from build123d import *

# Parameters (mm, degrees)
SKETCH1_W                        = 76.2
SKETCH1_H                        = 925.5125
BASE_FLANGE1_DEPTH               = 3.175
EDGE_FLANGE1_STRIP_W             = 20.32
EDGE_FLANGE1_STRIP_H             = 3.175
EDGE_FLANGE1_STRIP_CUT_DEPTH     = 925.5125
EDGE_FLANGE1_DEPTH               = 925.5125
EDGE_FLANGE2_STRIP_W             = 20.32
EDGE_FLANGE2_STRIP_H             = 3.175
EDGE_FLANGE2_STRIP_CUT_DEPTH     = 925.5125
EDGE_FLANGE2_DEPTH               = 925.5125
F_10_0_1935_DIAMETER_HOLE2_D     = 4.9149
F_10_0_1935_DIAMETER_HOLE1_D     = 4.9149
FILLET1_R                        = 3.175
O_0_316_DIAMETER_HOLE1_D         = 8.0264
F_27_64_0_42188_DIAMETER_HOLE1_D = 10.715752


# Sheet-metal steps are written as plain solids
with BuildPart() as part:
    # Sketch1 → Base-Flange1 (new body)
    with BuildSketch(Plane(origin=(0, 0, 0), x_dir=(0, 0, -1), z_dir=(1, 0, 0))):
        with Locations((38.1, 462.75625)):
            Rectangle(SKETCH1_W, SKETCH1_H)
    extrude(amount=-BASE_FLANGE1_DEPTH)

    # Edge-Flange1 strip (across the edge) → Edge-Flange1 strip cut (cut)
    with BuildSketch(Plane(origin=(-3.175, 0, 0), x_dir=(0, 0, -1), z_dir=(0, 1, 0))):
        with Locations((-6.35, -1.5875)):
            Rectangle(EDGE_FLANGE1_STRIP_W, EDGE_FLANGE1_STRIP_H)
    extrude(amount=EDGE_FLANGE1_STRIP_CUT_DEPTH, mode=Mode.SUBTRACT)

    # Edge-Flange1 section (across the edge) → Edge-Flange1 (add)
    with BuildSketch(Plane(origin=(-3.175, 0, 0), x_dir=(0, 0, -1), z_dir=(0, 1, 0))):
        with BuildLine():
            Line((-3.175, 3.81), (-3.175, 53.975))
            Line((-3.175, 53.975), (0, 53.975))
            Line((0, 53.975), (0, 3.81))
            ThreePointArc((0, 3.81), (1.115923164, 1.115923164), (3.81, 0))
            Line((3.81, 0), (3.81, -3.175))
            ThreePointArc((3.81, -3.175), (-1.129140867, -1.129140867), (-3.175, 3.81))
        make_face()
    extrude(amount=EDGE_FLANGE1_DEPTH)

    # Edge-Flange2 strip (across the edge) → Edge-Flange2 strip cut (cut)
    with BuildSketch(Plane(origin=(-3.175, 925.5125, -76.2), x_dir=(0, 0, 1), z_dir=(0, -1, 0))):
        with Locations((-6.35, -1.5875)):
            Rectangle(EDGE_FLANGE2_STRIP_W, EDGE_FLANGE2_STRIP_H)
    extrude(amount=EDGE_FLANGE2_STRIP_CUT_DEPTH, mode=Mode.SUBTRACT)

    # Edge-Flange2 section (across the edge) → Edge-Flange2 (add)
    with BuildSketch(Plane(origin=(-3.175, 925.5125, -76.2), x_dir=(0, 0, 1), z_dir=(0, -1, 0))):
        with BuildLine():
            Line((-3.175, 3.81), (-3.175, 53.975))
            Line((-3.175, 53.975), (0, 53.975))
            Line((0, 53.975), (0, 3.81))
            ThreePointArc((0, 3.81), (1.115923164, 1.115923164), (3.81, 0))
            Line((3.81, 0), (3.81, -3.175))
            ThreePointArc((3.81, -3.175), (-1.129140867, -1.129140867), (-3.175, 3.81))
        make_face()
    extrude(amount=EDGE_FLANGE2_DEPTH)

    # #10 (0.1935) Diameter Hole2 (through all)
    with Locations(Plane(origin=(0, 0, -79.375), x_dir=(-1, 0, 0), z_dir=(0, 0, -1))):
        with Locations((20.6375, 19.05), (46.0375, 19.05)):
            Hole(F_10_0_1935_DIAMETER_HOLE2_D / 2)

    # #10 (0.1935) Diameter Hole1 (through all)
    with Locations(Plane(origin=(0, 0, -79.375), x_dir=(-1, 0, 0), z_dir=(0, 0, -1))):
        with Locations((46.0375, 912.8125), (20.6375, 912.8125), (20.6375, 887.4125), (46.0375, 887.4125)):
            Hole(F_10_0_1935_DIAMETER_HOLE1_D / 2)

    # Fillet1
    fillet1_edges = [part.edges().sort_by_distance(p)[0] for p in [
        (-57.15, 0, 1.5875),
        (-57.15, 925.5125, 1.5875),
        (-57.15, 925.5125, -77.7875),
        (-57.15, 0, -77.7875),
    ]]
    fillet(fillet1_edges, radius=FILLET1_R)

    # O (0.316) Diameter Hole1 (through all)
    with Locations(Plane(origin=(0, 0, -79.375), x_dir=(-1, 0, 0), z_dir=(0, 0, -1))):
        with Locations((14.2875, 520.7), (14.2875, 444.5), (46.0375, 520.7), (46.0375, 444.5)):
            Hole(O_0_316_DIAMETER_HOLE1_D / 2)

    # 27/64 (0.42188) Diameter Hole1 (through all)
    with Locations(Plane.XY.offset(3.175)):
        with Locations((-41.275, 825.5), (-41.275, 781.05), (-41.275, 628.65), (-41.275, 584.2)):
            Hole(F_27_64_0_42188_DIAMETER_HOLE1_D / 2)


solid = part.part
Can you work these out from the model? Positions are in its coordinate system, mm. A direction names the side the tool comes from. Give positions to 0.01 mm unless a question says otherwise; leave off trailing zeros. Write each loop counter-clockwise with the first axis right and the second up, starting at its lowest first coordinate (ties: lowest second). Pieces come first, ordered by that corner, then holes. Notation, with made-up numbers: (31, -20.5) -> (46, -20.5) arc R24 ccw to (46, 14.5) -> close; hole circle Ø11 at (-3.5, -37). An arc over 180 degrees is marked (long way). Answer as a JSON object with one key per item and string values. Group by question number.
Item 1: Suppose I cut it at A-A (y = 290.5). Please give me the cut outline in (x, z) (3 decimals), plus the area to 3 significant figures.
Item 2: Suppose I cut it at B-B (z = -37). Please give me the cut outline in (x, y) (1 decimal), plus the area to 3 significant figures.
Item 3: I'm going to push flat-ended pins straight in: P1, Ø12, axis at y = 102.5, z = -41.5, coming from the -X side (3 decimals); P2, Ø9.5, axis at x = -41.275, y = 628.65, coming from the -Z side. Where does each tip first touch, or does it pass through?
Item 4: We'd pull the mould along Z, two halves only. Please class faces 3 (the face through (-3, 0, -38)), 4 (the face through (-32, 456, 3.175)), 5 (the face through (-3.175, 469, -38)), 6 (the face through (-32, 469, -79.375)): +Z half, -Z half, draft (parallel to the pull), parting line (faces both ways), or undercut.
Item 5: For faces 1 (the face through (-3, 925.512, -38)), 2 (the face through (-32, 456, 0)), which set-ups out of +Z, -Z, +X, -X, +Y, -Y let a thin tool reach every point of the face, with its end or its side?
Item 6: Please list where these lines run through material, in increasing order: line 1 (X direction, y = 444.5, z = 2.1); line 2 (Z direction, x = -20, y = 554.5) (3 decimals); line 3 (X direction, y = 324.5, z = -34) (3 decimals). Write a range as [from, to].
Findings:
{
 "1": {"outline": "(-57.15, -79.375) -> (-6.985, -79.375) arc R6.985 ccw to (0, -72.39) -> (0, -3.81) arc R6.985 ccw to (-6.985, 3.175) -> (-57.15, 3.175) -> (-57.15, 0) -> (-6.985, 0) arc R3.81 cw to (-3.175, -3.81) -> (-3.175, -72.39) arc R3.81 cw to (-6.985, -76.2) -> (-57.15, -76.2) -> close", "area": "590 mm²"},
 "2": {"outline": "(-3.2, 0) -> (0, 0) -> (0, 925.5) -> (-3.2, 925.5) -> close", "area": "2,940 mm²"},
 "3": {"P1": "stops at x = -3.175", "P2": "passes through"},
 "4": {"face 3": "draft", "face 4": "+Z half", "face 5": "undercut", "face 6": "-Z half"},
 "5": {"face 1": "+Z, -Z, +X, -X, +Y", "face 2": "-X, +Y, -Y"},
 "6": {"line 1": "x = [-57.15, -50.05], [-42.02, -18.3], [-10.27, -3.26]", "line 2": "z = [-79.375, -76.2], [0, 3.175]", "line 3": "x = [-3.175, 0]"}
}
